Can you work these out from the model? Positions are in its coordinate system, mm. Face numbers are marked on the shaded views. Round coordinates to 2 decimals unless told otherwise and drop trailing zeros. Loops run counter-clockwise (first coordinate to the right, second up) from the corner with the lowest first, then second, coordinate; pieces in that order, holes last.
from build123d import *

# Parameters (mm, degrees)
SKETCH1_R           = 7.5
BOSS_EXTRUDE1_DEPTH = 5
SKETCH3_R           = 1.5
CUT_EXTRUDE1_DEPTH  = 5


with BuildPart() as part:
    # Sketch1 → Boss-Extrude1 (new body)
    with BuildSketch(Plane.XY):
        Circle(SKETCH1_R)
    extrude(amount=BOSS_EXTRUDE1_DEPTH)

    # Sketch3 → Cut-Extrude1 (cut)
    with BuildSketch(Plane.XY.offset(5)):
        with Locations((0, 7.5)):
            Circle(SKETCH3_R)
        with Locations((4.408389392, 6.067627458)):
            Circle(SKETCH3_R)
        with Locations((7.132923872, 2.317627458)):
            Circle(SKETCH3_R)
        with Locations((7.132923872, -2.317627458)):
            Circle(SKETCH3_R)
        with Locations((4.408389392, -6.067627458)):
            Circle(SKETCH3_R)
        with Locations((0, -7.5)):
            Circle(SKETCH3_R)
        with Locations((-4.408389392, -6.067627458)):
            Circle(SKETCH3_R)
        with Locations((-7.132923872, -2.317627458)):
            Circle(SKETCH3_R)
        with Locations((-7.132923872, 2.317627458)):
            Circle(SKETCH3_R)
        with Locations((-4.408389392, 6.067627458)):
            Circle(SKETCH3_R)
    extrude(amount=-CUT_EXTRUDE1_DEPTH, mode=Mode.SUBTRACT)


solid = part.part
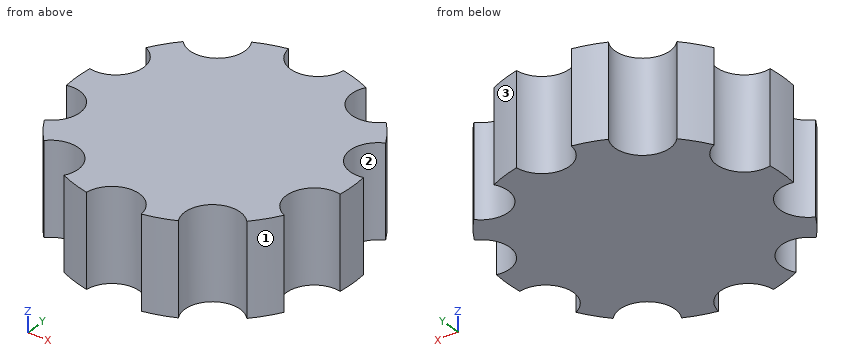
(1) If we section it at C-C, the plane x = -3.5: List the corners of the cut face in (y, z) for me.
Worked answers:
outline: (-4.87, 0) - (4.87, 0) - (4.87, 5) - (-4.87, 5) - close
(2) Will these pins go through, and if not, where does the flat tip stop? P1, Ø1, axis at x = -2, y = -4, coming from the -Z side; P2, Ø1.5, axis at y = -3.5, z = 1.5, coming from the +X side; P3, Ø1.5, axis at x = 3, z = 1.5, coming from the +Y side.
Worked answers:
P1: stops at z = 0
P2: stops at x = 6.53
P3: stops at y = 7.15
(3) If we section it at A-A, the plane y = 6.5: List the corners of the cut face in (x, z) for me, then the cut area to 3 significant figures.
Worked answers:
outline: (-2.97, 0) - (-1.12, 0) - (-1.12, 5) - (-2.97, 5) - close; (1.12, 0) - (2.97, 0) - (2.97, 5) - (1.12, 5) - close
area: 18.5 mm2
(4) If we section it at D-D, the plane y = -5.25: List the corners of the cut face in (x, z) for me, then the cut area to 3 significant figures.
Worked answers:
outline: (-3.15, 0) - (3.15, 0) - (3.15, 5) - (-3.15, 5) - close
area: 31.5 mm2
(5) If we mould it in two halves opening along Y, with no side actions, what happens to the marked faces 1, 2 and 3? For each: released by +Y, released by -Y, zero draft, split by the parting line, or undercut.
Worked answers:
face 1: released by -Y
face 2: undercut
face 3: released by +Y
(6) If I drill on line 1 (X direction, y = -6.5, z = 3.7); line 2 (X direction, y = -2.25, z = 4.7); line 3 (X direction, y = -6.25, z = 3.5), over which ranges is the centre line in solid material (lowest first)?
Worked answers:
line 1: x = -2.97 to -1.12, 1.12 to 2.97
line 2: x = -5.63 to 5.63
line 3: x = -2.92 to -0.83, 0.83 to 2.92
(7) If we section it at B-B, the plane z = 4.6: List the corners of the cut face in (x, y) for me, then the cut area to 3 significant figures.
Worked answers:
outline: (-7.45, -0.85) arc R1.5 cw to (-6.53, -3.69) arc R7.5 ccw to (-5.53, -5.07) arc R1.5 cw to (-3.11, -6.82) arc R7.5 ccw to (-1.49, -7.35) arc R1.5 cw to (1.49, -7.35) arc R7.5 ccw to (3.11, -6.82) arc R1.5 cw to (5.53, -5.07) arc R7.5 ccw to (6.53, -3.69) arc R1.5 cw to (7.45, -0.85) arc R7.5 ccw to (7.45, 0.85) arc R1.5 cw to (6.53, 3.69) arc R7.5 ccw to (5.53, 5.07) arc R1.5 cw to (3.11, 6.82) arc R7.5 ccw to (1.49, 7.35) arc R1.5 cw to (-1.49, 7.35) arc R7.5 ccw to (-3.11, 6.82) arc R1.5 cw to (-5.53, 5.07) arc R7.5 ccw to (-6.53, 3.69) arc R1.5 cw to (-7.45, 0.85) arc R7.5 ccw to start
area: 143 mm2
